```python
from build123d import *

# Parameters (mm, degrees)
F0_W     = 50.8
F0_H     = 101.6
F0_R     = 3.175
F0_R_2   = 2.032
F0_R_3   = 13.97
F1_DEPTH = 5.334
F2_R     = 3.175
F3_DEPTH = 25.4


with BuildPart() as f1:
    # F0 (on Top) → F1 (new body)
    with BuildSketch(Plane.XY):
        with Locations((-18.054181, 35.379866)):
            Rectangle(F0_W, F0_H)
        with Locations((-30.754181, 2.359866)):
            Circle(F0_R, mode=Mode.SUBTRACT)
        with Locations((-5.354181, 2.359866)):
            Circle(F0_R, mode=Mode.SUBTRACT)
        with Locations((-18.377712, 42.822066)):
            Circle(F0_R_2, mode=Mode.SUBTRACT)
        with Locations((-36.011981, 61.103397)):
            Circle(F0_R_2, mode=Mode.SUBTRACT)
        with Locations((-18.054181, 60.779866)):
            Circle(F0_R_3, mode=Mode.SUBTRACT)
        with Locations((-0.096381, 60.456336)):
            Circle(F0_R_2, mode=Mode.SUBTRACT)
        with Locations((-17.730651, 78.737666)):
            Circle(F0_R_2, mode=Mode.SUBTRACT)
    extrude(amount=F1_DEPTH)

    # F2 (on face) → F3 (cut)
    with BuildSketch(Plane(origin=(0, 0, 0), x_dir=(1, 0, 0), z_dir=(0, 0, -1))):
        with Locations((-5.354181, -2.359866)):
            Circle(F2_R)
        with Locations((-30.754181, -2.359866)):
            Circle(F2_R)
    extrude(amount=-F3_DEPTH, mode=Mode.SUBTRACT)


solid = f1.part
```
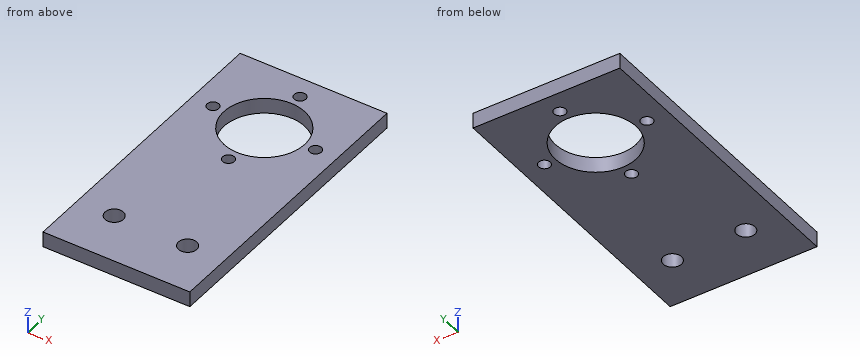
Could you check a few things on this model? Use its own coordinates, in mm. Coordinates: 2 decimals unless noted, no trailing zeros. Write each loop counter-clockwise with the first axis right and the second up, starting at its lowest first coordinate (ties: lowest second). Pieces come first, ordered by that corner, then holes. Notation, with made-up numbers: (-22.75, -31) - (14.25, -31) arc R26 ccw to (14.25, 1) - close; hole circle Ø10 at (72, 50). An arc over 180 degrees is marked (long way). Use a Markdown table: item, result.
Q1. Imagine slicing it at A-A (x = -18.5). List the corners of the cut face in (y, z) for me, and give its area (3 significant figures).
Geometry check:
| item | result |
|---|---|
| outline | (-15.42, 0) - (40.79, 0) - (40.79, 5.33) - (-15.42, 5.33) - close; (44.85, 0) - (46.82, 0) - (46.82, 5.33) - (44.85, 5.33) - close; (74.74, 0) - (76.86, 0) - (76.86, 5.33) - (74.74, 5.33) - close; (80.62, 0) - (86.18, 0) - (86.18, 5.33) - (80.62, 5.33) - close |
| area | 351 mm2 |
Q2. Imagine slicing it at D-D (y = 65.5). List the corners of the cut face in (x, z) for me, and give its area (3 significant figures).
Geometry check:
| item | result |
|---|---|
| outline | (-43.45, 0) - (-31.2, 0) - (-31.2, 5.33) - (-43.45, 5.33) - close; (-4.91, 0) - (7.35, 0) - (7.35, 5.33) - (-4.91, 5.33) - close |
| area | 131 mm2 |
Q3. Imagine slicing it at C-C (x = -1). List the corners of the cut face in (y, z) for me.
Geometry check:
| item | result |
|---|---|
| outline | (-15.42, 0) - (58.64, 0) - (58.64, 5.33) - (-15.42, 5.33) - close; (62.28, 0) - (86.18, 0) - (86.18, 5.33) - (62.28, 5.33) - close |
Q4. I'm going to push a flat-ended pin straight in: pin 1 Ø10 at (x, y) = (-36.5, 61) entering from +Z. Where does the tip first touch, or does it pass through?
Geometry check:
| item | result |
|---|---|
| pin 1 | stops at z = 5.33 |
Q5. Imagine slicing it at B-B (z = 1). List the corners of the cut face in (x, y) for me (3 decimals), and give its area (3 significant figures).
Geometry check:
| item | result |
|---|---|
| outline | (-43.454, -15.42) - (7.346, -15.42) - (7.346, 86.18) - (-43.454, 86.18) - close; hole circle Ø4.064 at (-36.012, 61.103); hole circle Ø6.35 at (-30.754, 2.36); hole circle Ø27.94 at (-18.054, 60.78); hole circle Ø4.064 at (-18.378, 42.822); hole circle Ø4.064 at (-17.731, 78.738); hole circle Ø6.35 at (-5.354, 2.36); hole circle Ø4.064 at (-0.096, 60.456) |
| area | 4,430 mm2 |
Q6. Please list where these lines run through material, in increasing order: L1, parallel to X at y = 79, z = 3.2; L2, parallel to Y at x = -19.5, z = 0.3; L3, parallel to Y at x = -17, z = 0.2.
Geometry check:
| item | result |
|---|---|
| L1 | x = -43.45 to -19.75, -15.72 to 7.35 |
| L2 | y = -15.42 to 41.13, 44.52 to 46.88, 74.67 to 77.74, 79.74 to 86.18 |
| L3 | y = -15.42 to 41.33, 44.32 to 46.85, 74.71 to 76.84, 80.63 to 86.18 |
